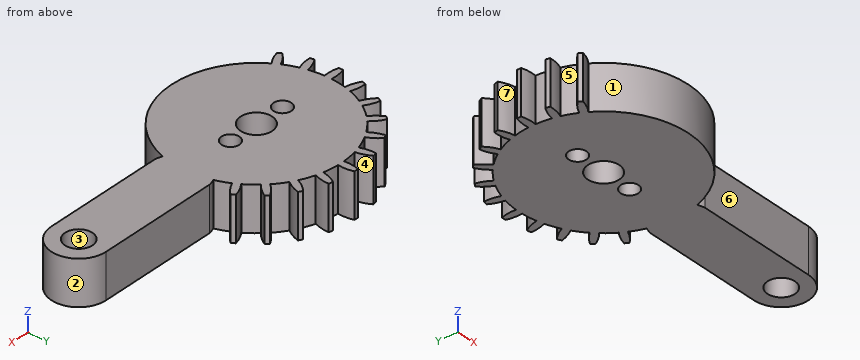
```python
from build123d import *

# Parameters (mm, degrees)
SKETCH1_R           = 1.75
SKETCH1_R_2         = 2
BOSS_EXTRUDE1_DEPTH = 6.5
SKETCH2_R           = 2.3
SKETCH2_R_2         = 1.3
CUT_EXTRUDE1_DEPTH  = 39.260284892


with BuildPart() as part:
    # Sketch1 → Boss-Extrude1 (new body)
    with BuildSketch(Plane.XY):
        with BuildLine():
            Line((0.31, 14.63), (-0.31, 14.63))
            ThreePointArc((-0.31, 14.63), (-0.532517386, 13.523085628), (-0.52, 12.394096377))
            ThreePointArc((-0.52, 12.394096377), (-1.619177414, 12.298873505), (-2.70554676, 12.106363687))
            ThreePointArc((-2.70554676, 12.106363687), (-2.985659813, 13.2001233), (-3.487085624, 14.211728743))
            Line((-3.487085624, 14.211728743), (-4.085959636, 14.051260935))
            ThreePointArc((-4.085959636, 14.051260935), (-4.014404405, 12.924472018), (-3.710109619, 11.837191881))
            ThreePointArc((-3.710109619, 11.837191881), (-4.747187978, 11.460725601), (-5.746714978, 10.993602319))
            ThreePointArc((-5.746714978, 10.993602319), (-6.30036923, 11.977594384), (-7.046532125, 12.824951657))
            Line((-7.046532125, 12.824951657), (-7.583467875, 12.514951657))
            ThreePointArc((-7.583467875, 12.514951657), (-7.222716398, 11.445076999), (-6.647381398, 10.473602319))
            ThreePointArc((-6.647381398, 10.473602319), (-7.551685527, 9.841548186), (-8.396254069, 9.131645121))
            ThreePointArc((-8.396254069, 9.131645121), (-9.185718896, 9.938812205), (-10.125769107, 10.564175311))
            Line((-10.125769107, 10.564175311), (-10.564175311, 10.125769107))
            ThreePointArc((-10.564175311, 10.125769107), (-9.938812205, 9.185718896), (-9.131645121, 8.396254069))
            ThreePointArc((-9.131645121, 8.396254069), (-9.841548186, 7.551685527), (-10.473602319, 6.647381398))
            ThreePointArc((-10.473602319, 6.647381398), (-11.445076999, 7.222716398), (-12.514951657, 7.583467875))
            Line((-12.514951657, 7.583467875), (-12.824951657, 7.046532125))
            ThreePointArc((-12.824951657, 7.046532125), (-11.977594384, 6.30036923), (-10.993602319, 5.746714978))
            ThreePointArc((-10.993602319, 5.746714978), (-11.460725601, 4.747187978), (-11.837191881, 3.710109619))
            ThreePointArc((-11.837191881, 3.710109619), (-12.924472018, 4.014404405), (-14.051260935, 4.085959636))
            Line((-14.051260935, 4.085959636), (-14.211728743, 3.487085624))
            ThreePointArc((-14.211728743, 3.487085624), (-13.2001233, 2.985659813), (-12.106363687, 2.70554676))
            ThreePointArc((-12.106363687, 2.70554676), (-12.298873505, 1.619177414), (-12.394096377, 0.52))
            ThreePointArc((-12.394096377, 0.52), (-13.523085628, 0.532517386), (-14.63, 0.31))
            Line((-14.63, 0.31), (-14.63, -0.31))
            ThreePointArc((-14.63, -0.31), (-13.523085628, -0.532517386), (-12.394096377, -0.52))
            ThreePointArc((-12.394096377, -0.52), (-12.298873505, -1.619177414), (-12.106363687, -2.70554676))
            ThreePointArc((-12.106363687, -2.70554676), (-13.2001233, -2.985659813), (-14.211728743, -3.487085624))
            Line((-14.211728743, -3.487085624), (-14.051260935, -4.085959636))
            ThreePointArc((-14.051260935, -4.085959636), (-12.924472018, -4.014404405), (-11.837191881, -3.710109619))
            ThreePointArc((-11.837191881, -3.710109619), (-11.460725601, -4.747187978), (-10.993602319, -5.746714978))
            ThreePointArc((-10.993602319, -5.746714978), (-11.977594384, -6.30036923), (-12.824951657, -7.046532125))
            Line((-12.824951657, -7.046532125), (-12.514951657, -7.583467875))
            ThreePointArc((-12.514951657, -7.583467875), (-11.445076999, -7.222716398), (-10.473602319, -6.647381398))
            ThreePointArc((-10.473602319, -6.647381398), (1.619177414, -12.298873505), (11.837191881, -3.710109619))
            ThreePointArc((11.837191881, -3.710109619), (12.333238692, -3.879500788), (12.84337176, -4))
            Line((12.84337176, -4), (30.75, -4))
            ThreePointArc((30.75, -4), (34.75, 0), (30.75, 4))
            Line((30.75, 4), (12.84337176, 4))
            ThreePointArc((12.84337176, 4), (12.333238692, 3.879500788), (11.837191881, 3.710109619))
            ThreePointArc((11.837191881, 3.710109619), (11.460725601, 4.747187978), (10.993602319, 5.746714978))
            ThreePointArc((10.993602319, 5.746714978), (11.977594384, 6.30036923), (12.824951657, 7.046532125))
            Line((12.824951657, 7.046532125), (12.514951657, 7.583467875))
            ThreePointArc((12.514951657, 7.583467875), (11.445076999, 7.222716398), (10.473602319, 6.647381398))
            ThreePointArc((10.473602319, 6.647381398), (9.841548186, 7.551685527), (9.131645121, 8.396254069))
            ThreePointArc((9.131645121, 8.396254069), (9.938812205, 9.185718896), (10.564175311, 10.125769107))
            Line((10.564175311, 10.125769107), (10.125769107, 10.564175311))
            ThreePointArc((10.125769107, 10.564175311), (9.185718896, 9.938812205), (8.396254069, 9.131645121))
            ThreePointArc((8.396254069, 9.131645121), (7.551685527, 9.841548186), (6.647381398, 10.473602319))
            ThreePointArc((6.647381398, 10.473602319), (7.222716398, 11.445076999), (7.583467875, 12.514951657))
            Line((7.583467875, 12.514951657), (7.046532125, 12.824951657))
            ThreePointArc((7.046532125, 12.824951657), (6.30036923, 11.977594384), (5.746714978, 10.993602319))
            ThreePointArc((5.746714978, 10.993602319), (4.747187978, 11.460725601), (3.710109619, 11.837191881))
            ThreePointArc((3.710109619, 11.837191881), (4.014404405, 12.924472018), (4.085959636, 14.051260935))
            Line((4.085959636, 14.051260935), (3.487085624, 14.211728743))
            ThreePointArc((3.487085624, 14.211728743), (2.985659813, 13.2001233), (2.70554676, 12.106363687))
            ThreePointArc((2.70554676, 12.106363687), (1.619177414, 12.298873505), (0.52, 12.394096377))
            ThreePointArc((0.52, 12.394096377), (0.532517386, 13.523085628), (0.31, 14.63))
        make_face()
        with Locations(Location((0, 0, 0), (0, 0, 180))):
            Circle(SKETCH1_R, mode=Mode.SUBTRACT)
        with Locations(Location((30.75, 0, 0), (0, 0, 180))):
            Circle(SKETCH1_R_2, mode=Mode.SUBTRACT)
    extrude(amount=BOSS_EXTRUDE1_DEPTH)

    # Sketch2 → Cut-Extrude1 (cut, through all)
    with BuildSketch(Plane.XY.offset(6.5)):
        Circle(SKETCH2_R)
        with Locations((4.5, 0)):
            Circle(SKETCH2_R_2)
        with Locations((-4.5, 0)):
            Circle(SKETCH2_R_2)
    extrude(amount=-CUT_EXTRUDE1_DEPTH, mode=Mode.SUBTRACT)


solid = part.part
```
Can you work these out from the model? Positions are in its coordinate system, mm. Face numbers are marked on the shaded views. A direction names the side the tool comes from. Give positions to 0.01 mm unless a question says otherwise; leave off trailing zeros. Loops run counter-clockwise (first coordinate to the right, second up) from the corner with the lowest first, then second, coordinate; pieces in that order, holes last. Notation, with made-up numbers: M 35,-28 L 68,-28 A27 ccw 68,-3 Z; hole C 29,81 d2. An arc over 180 degrees is marked long. Use one line per item in the form item = value. Start each with the question number.
(1) Thinking about a two-plate mould opening in Y: for the marked faces 1, 2 and 3, which applies, released by +Y, released by -Y, zero draft, split by the parting line, or undercut?
(2) I want a section at B-B, the plane x = 22. Write out the boundary of the cut face in (y, z).
(3) Please list where these lines run through material, in increasing order: line 1 (Y direction, x = 0, z = 3.5) (3 decimals); line 2 (Y direction, x = 30.75, z = 3.25); line 3 (X direction, y = 9.75, z = 1).
(4) On a 3-axis mill with a long thin cutter (end or side, diameter ignored), from which of +Z, -Z, +X, -X, +Y, -Y can I reach the whole of each face in a straight line? I mean the marked faces 4, 5, 6 and 7. Say none if no direction works.
(5) I want a section at A-A, the plane z = 5.25. State how many separate pieces and enclosed holes the cut face has, and give its area (3 significant figures).
(6) I'm going to push flat-ended pins straight in: P1, Ø3, axis at x = 19.5, z = 3, coming from the +Y side; P2, Ø4, axis at x = 15.5, y = -1, coming from the -Z side; P3, Ø1, axis at y = -4, z = 2, coming from the -X side; P4, Ø1.5, axis at y = 6.5, z = 2, coming from the -X side. Where does each tip first touch, or does it pass through?
(7) I want a section at C-C, the plane y = -4.75. Write out the boundary of the cut face in (x, z).
Worked out:
q1.face_1 = released by -Y
q1.face_2 = split by the parting line
q1.face_3 = undercut
q2.outline = M -4,0 L 4,0 L 4,6.5 L -4,6.5 Z
q3.line_1 = -12.405 to -2.3, 2.3 to 14.63
q3.line_2 = -4 to -2, 2 to 4
q3.line_3 = -10.35 to -8.97, -7.67 to 7.67, 8.97 to 10.35
q4.face_4 = +Z, -Z, +Y
q4.face_5 = +Z, -Z
q4.face_6 = +Z, -Z, +X, -Y
q4.face_7 = +Z, -Z, -X
q5.separate_pieces = 1
q5.enclosed_holes = 4
q5.area = 646 mm²
q6.P1 = 4
q6.P2 = 0
q6.P3 = -14.21
q6.P4 = -12.82
q7.outline = M -11.46,0 L 11.46,0 L 11.46,6.5 L -11.46,6.5 Z
